Here's how the part is built. I have some questions about the finished solid (model axes, mm). Give positions to 0.01 mm unless a question says otherwise; leave off trailing zeros. Loops run counter-clockwise (first coordinate to the right, second up) from the corner with the lowest first, then second, coordinate; pieces in that order, holes last. Notation, with made-up numbers: M 31,39.25 L 37,39.25 A19 ccw 37,57.25 Z; hole C -17,59.5 d6. An arc over 180 degrees is marked long. Answer as CSV lines item,"result". Start each with the question number.
Item 1: I want a section at D-D on x = 24. List the corners of the cut face in (y, z) for me.
Item 2: I want a section at C-C on z = -75.5. List the corners of the cut face in (x, y) for me, plus the area to 3 significant figures.
Item 3: If we mould it in two halves opening along Z, with no side actions, what happens to faces 1 (the flat face through (-129, 0, -123)), 2 (the flat face through (-237.34, -9.86, -104.57)), 3 (the cylindrical face through (-151.04, -9.86, 3.24))? For each: released by +Z, released by -Z, zero draft, split by the parting line, or undercut.
Item 4: I want a section at A-A on x = -121. List the corners of the cut face in (y, z) for me, plus the area to 3 significant figures.
Item 5: If I drill on line 1 along Z through (x, y) = (-125, -5.5); line 2 along Z through (x, y) = (-125.5, -5.5); line 3 along X through (y, z) = (-1.25, 0), over which ranges is the centre line in solid material (lowest first)? Write a range as from..to.
Item 6: Will these pins go through, and if not, where does the flat tip stop? P1, Ø4, axis at y = -17, z = -1.5, coming from the +X side; P2, Ø12, axis at x = -70, y = -6, coming from the +Z side; P3, Ø1, axis at x = 18, y = -7.5, coming from the +Z side.
Item 7: I want a section at B-B on y = -7.25. List the corners of the cut face in (x, z) for me.
from build123d import *

# Parameters (mm, degrees)
F0_R     = 25
F1_DEPTH = 20


with BuildPart() as f1:
    # F0 (on Front) → F1 (new body)
    with BuildSketch(Plane.XZ):
        with BuildLine():
            Line((-126.065396, -237.863924), (53.934604, -237.863924))
            Line((53.934604, -237.863924), (-81.624864, 25.049808))
            ThreePointArc((-81.624864, 25.049808), (-100.043162, 44.830845), (-126.065396, 52.136076))
            ThreePointArc((-126.065396, 52.136076), (-152.087631, 44.830845), (-170.505928, 25.049808))
            Line((-170.505928, 25.049808), (-306.065396, -237.863924))
            Line((-306.065396, -237.863924), (-126.065396, -237.863924))
        make_face()
        with Locations((-126.065396, 2.136076)):
            Circle(F0_R, mode=Mode.SUBTRACT)
    extrude(amount=F1_DEPTH)


solid = f1.part
Result:
1,outline,"M -20,-237.86 L 0,-237.86 L 0,-179.81 L -20,-179.81 Z"
2,outline,"M -222.35,-20 L -29.78,-20 L -29.78,0 L -222.35,0 Z"
2,area,"3,850 mm^2"
3,face 1,"zero draft"
3,face 2,"released by +Z"
3,face 3,"undercut"
4,outline,"M -20,-237.86 L 0,-237.86 L 0,-22.35 L -20,-22.35 Z; M -20,26.62 L 0,26.62 L 0,51.88 L -20,51.88 Z"
4,area,"4,820 mm^2"
5,line 1,"-237.86..-22.84, 27.11..52.12"
5,line 2,"-237.86..-22.86, 27.13..52.13"
5,line 3,"-183.42..-150.97, -101.16..-68.71"
6,P1,"x = -66.9"
6,P2,"z = 14.14"
6,P3,"z = -167.2"
7,outline,"M -306.07,-237.86 L 53.93,-237.86 L -81.62,25.05 A50 ccw -126.07,52.14 A50 ccw -170.51,25.05 Z; hole C -126.07,2.14 d50"
